```python
from build123d import *

# Parameters (mm, degrees)
BOSS_EXTRUDE1_DEPTH = 9
CUT_EXTRUDE1_DEPTH  = 26
BOSS_EXTRUDE2_DEPTH = 18
LPATTERN1_COUNT     = 6
LPATTERN1_PITCH     = 6
FILLET1_R           = 6
FILLET2_R           = 6
FILLET3_R           = 6
SKETCH4_R           = 1.5
CUT_EXTRUDE2_DEPTH  = 88.522155905
CUT_EXTRUDE3_DEPTH  = 9
SKETCH6_R           = 1.75
BOSS_EXTRUDE3_DEPTH = 2
SKETCH7_R           = 1.25
CUT_EXTRUDE4_DEPTH  = 0.5
CUT_EXTRUDE5_DEPTH  = 1


with BuildPart() as part:
    # Sketch1 → Boss-Extrude1 (new, symmetric)
    with BuildSketch(Plane(origin=(0, 0, 0), x_dir=(1, 0, 0), z_dir=(0, 1, 0))):
        with BuildLine():
            Line((2.514105873, -21.575108952), (-33.455759115, 38.476275817))
            Line((-33.455759115, 38.476275817), (-12.667369645, 50.469726664))
            Line((-12.667369645, 50.469726664), (11.092875126, -16.436556811))
            Line((11.092875126, -16.436556811), (21.575489497, -19.497759324))
            Line((21.575489497, -19.497759324), (27.289214074, -11.555417826))
            ThreePointArc((27.289214074, -11.555417826), (35.663709394, -10.188732731), (37.030394489, -18.56322805))
            Line((37.030394489, -18.56322805), (31.190552636, -26.680878395))
            Line((31.190552636, -26.680878395), (31.190552636, -76.680878395))
            Line((31.190552636, -76.680878395), (20.190552636, -76.680878395))
            Line((20.190552636, -76.680878395), (20.190552636, -69.680878395))
            Line((20.190552636, -69.680878395), (8.563166422, -42.02579044))
            Line((8.563166422, -42.02579044), (-1.775278753, -34.144385023))
            Line((-1.775278753, -34.144385023), (-1.775278753, -24.144385023))
            Line((-1.775278753, -24.144385023), (2.514105873, -21.575108952))
        make_face()
    extrude(amount=BOSS_EXTRUDE1_DEPTH, both=True)

    # Sketch2 → Cut-Extrude1 (cut)
    with BuildSketch(Plane(origin=(0, 9, 0), x_dir=(1, 0, 0), z_dir=(0, 1, 0))):
        Polygon((12.928109305, -44.071308637), (27.928109305, -44.071308637), (27.928109305, -69.071308637), align=None)
    extrude(amount=-CUT_EXTRUDE1_DEPTH, mode=Mode.SUBTRACT)

    # Sketch3 → Boss-Extrude2 (add)
    with BuildSketch(Plane(origin=(0, 9, 0), x_dir=(1, 0, 0), z_dir=(0, 1, 0))):
        Polygon((31.190552636, -69.680878395), (31.190552636, -65.680878395), (35.190552636, -67.680878395), align=None)
    boss_extrude2 = extrude(amount=-BOSS_EXTRUDE2_DEPTH)

    # LPattern1: Boss-Extrude2 ×6
    with Locations(*[(0, 0, -i * LPATTERN1_PITCH) for i in range(1, LPATTERN1_COUNT)]):
        add(boss_extrude2)

    # Fillet1
    fillet1_edges = [part.edges().sort_by_distance(p)[0] for p in [
        (-33.455759115, 0, -38.476275817),
        (-12.667369645, 0, -50.469726664),
    ]]
    fillet(fillet1_edges, radius=FILLET1_R)

    # Fillet2
    fillet2_edges = [part.edges().sort_by_distance(p)[0] for p in [
        (-1.775278753, 0, 34.144385023),
        (-1.775278753, 0, 24.144385023),
    ]]
    fillet(fillet2_edges, radius=FILLET2_R)

    # Fillet3
    fillet3_edges = [part.edges().sort_by_distance(p)[0] for p in [
        (20.190552636, 0, 76.680878395),
    ]]
    fillet(fillet3_edges, radius=FILLET3_R)

    # Sketch4 → Cut-Extrude2 (cut, through all)
    with BuildSketch(Plane(origin=(0, 9, 0), x_dir=(1, 0, 0), z_dir=(0, 1, 0))):
        with Locations(Location((-25.174418311, 36.32708835, 0), (0, 0, 270))):
            Circle(SKETCH4_R)
    extrude(amount=-CUT_EXTRUDE2_DEPTH, mode=Mode.SUBTRACT)

    # Sketch5 → Cut-Extrude3 (cut)
    with BuildSketch(Plane(origin=(-7.738353784, 0, 3.25353614), x_dir=(0.38757954045785686, 0, 0.9218362651894731), z_dir=(-0.921836265189473, 0, 0.3875795404578568))):
        Polygon((49.059805807, 6), (49.059805807, -6), (70.059805807, -8.207927909), (70.059805807, 3.792072091), align=None)
    extrude(amount=-CUT_EXTRUDE3_DEPTH, mode=Mode.SUBTRACT)

    # Sketch6 → Boss-Extrude3 (add)
    with BuildSketch(Plane(origin=(0, 9, 0), x_dir=(1, 0, 0), z_dir=(0, 1, 0))):
        with Locations(Location((32.159804282, -15.059322938, 0), (0, 0, 270))):
            Circle(SKETCH6_R)
        with Locations(Location((4.224721247, -31.173767393, 0), (0, 0, 270))):
            Circle(SKETCH6_R)
    boss_extrude3 = extrude(amount=BOSS_EXTRUDE3_DEPTH)

    # Sketch7 → Cut-Extrude4 (cut)
    with BuildSketch(Plane(origin=(0, 11, 0), x_dir=(1, 0, 0), z_dir=(0, 1, 0))):
        with Locations(Location((4.224721247, -31.173767393, 0), (0, 0, 270))):
            Circle(SKETCH7_R)
        with Locations(Location((32.159804282, -15.059322938, 0), (0, 0, 270))):
            Circle(SKETCH7_R)
    cut_extrude4 = extrude(amount=-CUT_EXTRUDE4_DEPTH, mode=Mode.SUBTRACT)

    # Sketch8 → Cut-Extrude5 (cut)
    with BuildSketch(Plane(origin=(0, 9, 0), x_dir=(1, 0, 0), z_dir=(0, 1, 0))):
        with BuildLine():
            Line((-14.087027859, 31.922607918), (7.364953265, -12.596019576))
            ThreePointArc((7.364953265, -12.596019576), (6.240093161, -15.813119473), (3.022993263, -14.688259369))
            Line((3.022993263, -14.688259369), (-18.428987861, 29.830368124))
            ThreePointArc((-18.428987861, 29.830368124), (-17.304127757, 33.047468022), (-14.087027859, 31.922607918))
        make_face()
    cut_extrude5 = extrude(amount=-CUT_EXTRUDE5_DEPTH, mode=Mode.SUBTRACT)

    # Mirror1: Boss-Extrude3, Cut-Extrude4, Cut-Extrude5 across plane
    add(boss_extrude3.mirror(Plane.ZX))
    add(cut_extrude4.mirror(Plane.ZX), mode=Mode.SUBTRACT)
    add(cut_extrude5.mirror(Plane.ZX), mode=Mode.SUBTRACT)


solid = part.part
```
Can you work these out from the model? Positions are in its coordinate system, mm. A direction names the side the tool comes from. Give positions to 0.01 mm unless a question says otherwise; leave off trailing zeros. Loops run counter-clockwise (first coordinate to the right, second up) from the corner with the lowest first, then second, coordinate; pieces in that order, holes last. Notation, with made-up numbers: M 41,0 L 52,0 A28 cw 52,39 Z; hole C 65.5,-33 d5. An arc over 180 degrees is marked long. Use CSV: the item, a comma, the result in double quotes. Start each with the question number.
1. Imagine slicing it at B-B, the plane x = -8.5. Write out the boundary of the cut face in (y, z), plus the area to 3 significant figures.
2. For P1, Ø1.5, axis at x = -21, y = -6.5, coming from the +Z side; P2, Ø7.5, axis at y = 1.5, z = 74.5, coming from the +X side; P3, Ø12, axis at y = -3, z = 60.5, coming from the +X side, each with a flat end and sliding along its axis, tell me the tip position at first contact or that it passes through.
3. On a 3-axis mill with a long thin cutter (end or side, diameter ignored), from which of +Z, -Z, +X, -X, +Y, -Y can I reach the whole of each face in a straight line? I mean faces 1 (the face through (3.55, 9.99, 32.79)), 2 (the face through (17.66, -7.09, 57.03)), 3 (the face through (4, -10.5, 31)), 4 (the face through (33.163, 0.126, 36.667)), 5 (the face through (14.46, 6.13, 56.05)). Say none if no direction works.
4. If we mould it in two halves opening along X, with no side actions, what happens to faces 6 (the face through (-1.17, 0.13, 33.8)), 7 (the face through (33.219, 0.126, 62.667)), 8 (the face through (-24.16, 0.13, -37.43))? For each: released by +X, released by -X, zero draft, split by the parting line, or undercut.
5. If I drill on L1, parallel to X at y = 0.5, z = 59.5; L2, parallel to X at y = 8.25, z = 7; L3, parallel to X at y = 7.5, z = 15, over which ranges is the centre line in solid material (lowest first)?
6. Imagine slicing it at A-A, the plane z = -10. Write out the boundary of the cut face in (x, y), plus the area to 3 significant figures.
Response values:
1,outline,"M -9,-38.73 L 9,-38.73 L 9,-20.33 L 8,-20.33 L 8,-9.23 L 9,-9.23 L 9,3.19 L -9,3.19 L -9,-9.23 L -8,-9.23 L -8,-20.33 L -9,-20.33 Z"
1,area,"732 mm^2"
2,P1,"z = -16.43"
2,P2,"x = 31.19"
2,P3,"x = 35.19"
3,face 1,"+Y"
3,face 2,"none"
3,face 3,"-Y"
3,face 4,"+X, +Y, -Y"
3,face 5,"+Z, -X, +Y, -Y"
4,face 6,"released by -X"
4,face 7,"released by +X"
4,face 8,"undercut"
5,L1,"27.93 to 31.19"
5,L2,"-6.22 to -0.68, 4.67 to 7.74"
5,L3,"-1.42 to 10.58, 24.81 to 38.16"
6,outline,"M -16.4,-9 L -8.87,-9 L -8.87,-8 L -3.52,-8 L -3.52,-9 L 1.7,-9 L 1.7,9 L -3.52,9 L -3.52,8 L -8.87,8 L -8.87,9 L -16.4,9 Z"
6,area,"315 mm^2"
